Verification items for the finished model (mm, model axes). Face numbers are marked on the shaded views. A direction names the side the tool comes from. Round coordinates to 2 decimals unless told otherwise and drop trailing zeros. Order: outer loops, then holes, each group sorted by start corner. A loop starts at its lowest first (then second) coordinate and runs counter-clockwise, first axis right, second up. Notation, with made-up numbers: (-24.5, -27.75) -> (7.5, -27.75) arc R17 ccw to (7.5, 4.25) -> close; hole circle Ø10 at (31, -26). An arc over 180 degrees is marked (long way). Return JSON: item names as keys, results as strings. Group by question number.
Item 1: Scan lines: probe 1 along Z at (x, y) = (42, -13); probe 2 along Y at (x, z) = (158, 2.5); probe 3 along Y at (x, z) = (94, 5.25). Record each from-to range of solid material in increasing order. Write a range as from..to.
Item 2: Sectioned sample at B-B on y = -70.5. Record the cut outline in (x, z), plus the area to 3 significant figures.
Item 3: Depth check by flat-ended pin: pin 1 Ø1.5 at (x, z) = (148, 7) entering from +Y; pin 2 Ø4 at (x, y) = (71.5, -51.5) entering from +Z; pin 3 Ø4 at (x, z) = (57.5, 4) entering from +Y. Enter the tip coordinate at first touch or a pass-through.
Item 4: Access from +Z, -Z, +X, -X, +Y, -Y to the whole of each face (thin tool, end or side, straight path). Record for the marked faces 1 and 2.
Item 5: Sectioned sample at D-D on y = -31. Record the cut outline in (x, z).
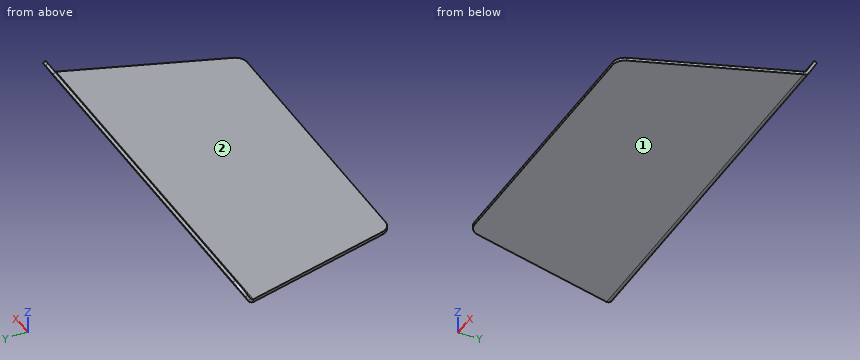
Autodesk Inventor part; units mm, degrees
ref_plane "YZ Plane" through (0, 0, 0) normal (1, 0, 0) x (0, 1, 0)
ref_plane "XZ Plane" through (0, 0, 0) normal (0, 1, 0) x (-1, 0, 0)
ref_plane "XY Plane" through (0, 0, 0) normal (0, 0, 1) x (1, 0, 0)
sketch "Sketch1" plane through (0, 0, 0) normal (0, 0, 1) x (1, 0, 0)
  line L0 (26.2341, -88.9) -> (159.0469, -88.9)
  circle A0 centre (190.5233, -0.0123) radius 2.1844
  arc A1 (193.5393, 5.5758) -> (190.4426, 6.3372) centre (190.5233, -0.0123) ccw
  line L1 (165.0634, -0.0075) -> (177.7634, -0.0075) construction
  line L2 (190.4426, 6.3372) -> (182.7263, 6.3372)
  line L3 (182.7263, 6.3372) -> (-0.0289, 6.3363)
  line L4 (193.5393, 5.5758) -> (193.5393, -6.3491)
  line L5 (193.5393, -6.3491) -> (165.014, -84.7218)
  arc A2 (159.0469, -88.9) -> (165.014, -84.7218) centre (159.0469, -82.55) ccw
  circle A3 centre (-0.0565, -0.0137) radius 2.1845
  arc A4 (-0.0289, 6.3363) -> (-6.4066, -0.0138) centre (-0.0565, -0.0137) ccw
  line L6 (26.2341, -88.9) -> (18.6122, -88.9)
  arc A5 (12.4412, -84.0472) -> (18.6122, -88.9) centre (18.6122, -82.55) ccw
  line L7 (193.5393, -6.3491) -> (-6.4065, -6.3491)
  line L8 (-6.4066, -0.0137) -> (-6.4065, -6.3637)
  line L9 (-6.4065, -6.3637) -> (12.4412, -84.0472)
  point P0 (157.3842, 6.3371)
  point P1 (13.5341, -88.9)
  dimension "d9" = 4.3688
  dimension "d26" = 6.35
  dimension "d29" = 12.7
  dimension "d30" = 6.35
extrude "Extrusion1" add sketch "Sketch1" along normal blind 1.5875
bend part "Bend Part1" radius 3.175 angle 60 line through (193.5393, -6.3491, 0) along (-1, 0, 0) centre toward (0, 0, 1) moving side (0, 1, 0) both sides no
properties part number "wing_wedge" material "Acetal Resin, White"
Recorded:
{
 "1": {"probe 1": "0..1.59", "probe 2": "-4.91..-3.07", "probe 3": "-3.32..-1.48"},
 "2": {"outline": "(9.15, 0) -> (170.19, 0) -> (170.19, 1.59) -> (9.15, 1.59) -> close", "area": "256 mm²"},
 "3": {"pin 1": "y = -0.04", "pin 2": "z = 1.59", "pin 3": "y = -1.05"},
 "4": {"face 1": "-Z, +X, -X, +Y, -Y", "face 2": "+Z, +X, -X, -Y"},
 "5": {"outline": "(-0.43, 0) -> (184.57, 0) -> (184.57, 1.59) -> (-0.43, 1.59) -> close"}
}
